Input: part model. Units: mm. Frame: model coordinates. Give positions to 0.01 mm unless a question says otherwise; leave off trailing zeros. Write each loop counter-clockwise with the first axis right and the second up, starting at its lowest first coordinate (ties: lowest second). Pieces come first, ordered by that corner, then holes. Notation, with made-up numbers: (-9.75, 49) - (-2.75, 49) arc R10 cw to (-2.75, 62) - close; hole circle Ø5 at (73.25, 21.25). An arc over 180 degrees is marked (long way). Answer as CSV lines item,"result". Start each with the question number.
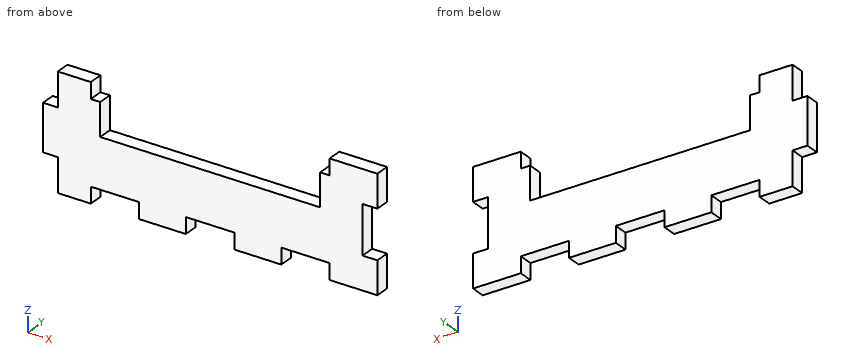
from build123d import *

# Parameters (mm, degrees)
BOSS_EXTRUDE1_DEPTH = 3


with BuildPart() as part:
    # Sketch3 → Boss-Extrude1 (new body)
    with BuildSketch(Plane(origin=(0, 0, 0), x_dir=(1, 0, 0), z_dir=(0, 1, 0))):
        Polygon((-35.058452488, 17.4), (-35.058452488, 7.6), (-31.958452488, 7.6), (-31.958452488, 0.5), (-25.041751777, 0.5), (-25.041751777, 3.85), (-23.058452488, 3.85), (-23.058452488, 10.75), (23.058452488, 10.75), (23.058452488, 3.85), (25.041751777, 3.85), (25.041751777, 0.5), (35.058452488, 0.5), (35.058452488, 7.4), (31.958452488, 7.4), (31.958452488, 17.6), (35.058452488, 17.6), (35.058452488, 24.5), (25.041751777, 24.5), (25.041751777, 21.15), (14.925051066, 21.15), (14.925051066, 24.5), (5.108350355, 24.5), (5.108350355, 21.15), (-5.108350355, 21.15), (-5.108350355, 24.5), (-14.925051066, 24.5), (-14.925051066, 21.15), (-25.041751777, 21.15), (-25.041751777, 24.5), (-31.958452488, 24.5), (-31.958452488, 17.4), align=None)
    extrude(amount=-BOSS_EXTRUDE1_DEPTH)


solid = part.part
1) Cut plane A-A on z = -2. Output: boundary loops of the cut face in (x, y).
2) Material intervals for line 1 (X direction, y = -2, z = -22.75); line 2 (X direction, y = -1.65, z = -2.25); line 3 (X direction, y = -2.7, z = -7), sorted ascending. Write a range as from..to.
3) Cut plane D-D on x = -10.5. Output: boundary loops of the cut face in (y, z).
4) Cut plane C-C on z = -6.5. Output: boundary loops of the cut face in (x, y).
5) Contact query for flat-ended pins moving along their axis: P1, Ø1.5, axis at y = -1.5, z = -13.5, coming from the +X side; P2, Ø0.6, axis at x = 24, y = -2, coming from the +Z side; P3, Ø1.5, axis at y = -2, z = -6.5, coming from the -X side. Output: stop coordinate, or through.
Numbers:
1,outline,"(-31.96, -3) - (-25.04, -3) - (-25.04, 0) - (-31.96, 0) - close; (25.04, -3) - (35.06, -3) - (35.06, 0) - (25.04, 0) - close"
2,line 1,"x = -31.96..-25.04, -14.93..-5.11, 5.11..14.93, 25.04..35.06"
2,line 2,"x = -31.96..-25.04, 25.04..35.06"
2,line 3,"x = -31.96..-23.06, 23.06..35.06"
3,outline,"(-3, -24.5) - (0, -24.5) - (0, -10.75) - (-3, -10.75) - close"
4,outline,"(-31.96, -3) - (-23.06, -3) - (-23.06, 0) - (-31.96, 0) - close; (23.06, -3) - (35.06, -3) - (35.06, 0) - (23.06, 0) - close"
5,P1,"stops at x = 31.96"
5,P2,"stops at z = -3.85"
5,P3,"stops at x = -31.96"
